Verification items for the finished model (mm, model axes). A direction names the side the tool comes from. Round coordinates to 2 decimals unless told otherwise and drop trailing zeros. Loops run counter-clockwise (first coordinate to the right, second up) from the corner with the lowest first, then second, coordinate; pieces in that order, holes last. Notation, with made-up numbers: (-12, 49) -> (14, 49) arc R26 ccw to (14, 82) -> close; hole circle Ø8 at (34.5, -13.5). An arc over 180 degrees is marked (long way). Write item = value, one per line.
```python
from build123d import *

# Parameters (mm, degrees)
F1_R     = 51.572415
F2_DEPTH = 25
F0_R     = 29.127335
F3_DEPTH = 73.050177
F4_SIZE  = 5
F5_R     = 15
F6_W     = 56.66241
F6_H     = 47.336116
F7_DEPTH = 91.210647


with BuildPart() as f2:
    # F1 (on Front) → F2 (new body)
    with BuildSketch(Plane.XZ):
        Circle(F1_R)
    extrude(amount=F2_DEPTH)

    # F0 (on Front) → F3 (join)
    with BuildSketch(Plane.XZ):
        Circle(F0_R)
    extrude(amount=F3_DEPTH)

    # F4
    f4_edges = [f2.edges().sort_by_distance(p)[0] for p in [
        (-29.127335, -73.050177, 0),
    ]]
    chamfer(f4_edges, length=F4_SIZE)

    # F5
    f5_edges = [f2.edges().sort_by_distance(p)[0] for p in [
        (-51.572415, -25, 0),
    ]]
    fillet(f5_edges, radius=F5_R)

    # F6 (on face) → F7 (cut)
    with BuildSketch(Plane(origin=(0, 0, 0), x_dir=(-1, 0, 0), z_dir=(0, 1, 0))):
        Rectangle(F6_W, F6_H)
    extrude(amount=-F7_DEPTH, mode=Mode.SUBTRACT)


solid = f2.part
```
(1) Sectioned sample at D-D, the plane y = -7. Record the cut outline in (x, z).
Filled sheet:
outline = circle Ø103.14 at (0, 0); hole (-28.33, -23.67) -> (28.33, -23.67) -> (28.33, 23.67) -> (-28.33, 23.67) -> close
(2) Draft check along Z on faces 1 (the face through (-0.254, -46.224, -29.126)), 2 (the face through (0.232, -70.585, 26.591)), 3 (the face through (0, -28, 23.668)). Enter one of: released by +Z, released by -Z, zero draft, split by the parting line, or undercut.
Filled sheet:
face_1 = released by -Z
face_2 = released by +Z
face_3 = undercut
(3) Go/stop test with flat-tipped pins: pin 1 Ø4 at (x, z) = (32, 8) entering from -Y; pin 2 Ø1 at (x, y) = (-36.5, -13.5) entering from +Z; pin 3 Ø6.5 at (x, z) = (0.5, -28) entering from -Y; pin 4 Ø6 at (y, z) = (-63.5, -19) entering from -X. Record where each tip stops, or that it passes through.
Filled sheet:
pin_1 = -25
pin_2 = 36.37
pin_3 = -72.42
pin_4 = through
(4) Material ranges on probe 1 along X at (y, z) = (-36, 0.5); probe 2 along Z at (x, y) = (1, -67); probe 3 along Z at (x, y) = (6, -31), recorded low to high. Write a range as from..to.
Filled sheet:
probe_1 = -29.12..-28.33, 28.33..29.12
probe_2 = -29.11..-23.67, 23.67..29.11
probe_3 = -28.5..-23.67, 23.67..28.5
(5) Sectioned sample at C-C, the plane x = 0. Record the cut outline in (y, z), and give its area (3 significant figures).
Filled sheet:
outline = (-73.05, -24.13) -> (-68.05, -29.13) -> (-25, -29.13) -> (-25, -36.57) arc R15 ccw to (-10, -51.57) -> (0, -51.57) -> (0, -23.67) -> (-73.05, -23.67) -> close; (-73.05, 23.67) -> (0, 23.67) -> (0, 51.57) -> (-10, 51.57) arc R15 ccw to (-25, 36.57) -> (-25, 29.13) -> (-68.05, 29.13) -> (-73.05, 24.13) -> close
area = 1,800 mm2
(6) Sectioned sample at A-A, the plane z = 0. Record the cut outline in (x, y).
Filled sheet:
outline = (-51.57, -10) arc R15 ccw to (-36.57, -25) -> (-29.13, -25) -> (-29.13, -68.05) -> (-28.33, -68.85) -> (-28.33, 0) -> (-51.57, 0) -> close; (28.33, -68.85) -> (29.13, -68.05) -> (29.13, -25) -> (36.57, -25) arc R15 ccw to (51.57, -10) -> (51.57, 0) -> (28.33, 0) -> close
(7) Set-up check for faces 4 (the face through (-29.127, -46.224, 0.096)), 5 (the face through (28.331, -26, 0)), 6 (the face through (0, -25, 30)): record each of +Z, -Z, +X, -X, +Y, -Y from which the full face is reachable in a straight line by a thin tool's end or side.
Filled sheet:
face_4 = -X, -Y
face_5 = +Y, -Y
face_6 = +Z, -Y
(8) Sectioned sample at B-B, the plane y = -42.5. Record the cut outline in (x, z), and give its area (3 significant figures).
Filled sheet:
outline = (-28.33, -6.76) -> (-28.33, 6.76) arc R29.13 ccw to start; (-16.98, -23.67) arc R29.13 ccw to (16.98, -23.67) -> close; (-16.98, 23.67) -> (16.98, 23.67) arc R29.13 ccw to start; (28.33, -6.76) arc R29.13 ccw to (28.33, 6.76) -> close
area = 267 mm2
